Geometry: final body of the model. Coordinates: model frame, mm. Face numbers are marked on the shaded views. A direction names the side the tool comes from. Give positions to 0.01 mm unless a question says otherwise; leave off trailing zeros. Order: outer loops, then holes, each group sorted by start corner. A loop starts at its lowest first (then second) coordinate and runs counter-clockwise, first axis right, second up. Notation, with made-up numbers: (74, -12) -> (107, -12) arc R22 ccw to (107, 20) -> close; hole circle Ø6 at (29, -26). An arc over 180 degrees is marked (long way). Answer in a Markdown table with one row per item. Add a question column.
Q1. Contact query for flat-ended pins moving along their axis: P1, Ø6.5, axis at y = -132, z = 4.5, coming from the -X side; P2, Ø6, axis at x = 420.5, z = -61.5, coming from the +Y side; P3, Ø9, axis at y = -115, z = 4.5, coming from the +X side. Output: stop coordinate, or through.
Q2. Cut plane A-A on z = -26. Return the cut outline in (x, y).
Q3. Cut plane D-D on y = -129.5. Return the cut outline in (x, z), and give its area (3 significant figures).
Q4. Cut plane B-B on x = 380. Return the cut outline in (y, z), and give its area (3 significant figures).
Q5. Set-up query: the marked faces 1 and 2. Return all of +Z, -Z, +X, -X, +Y, -Y with unobstructed straight access to the full face (end or side cutting, diameter ignored); none if empty.
Q6. Cut plane C-C on y = -81. Return the cut outline in (x, z), and give its area (3 significant figures).
Q7. Line query: line 1 along X through (y, z) = (-82, -13); line 2 along Y through (x, z) = (322, -4.5); line 3 along Z through (x, y) = (51.5, -206.5). Output: solid intervals per line, ascending. Write a range as from..to.
Q8. Pull-direction query (Y, two-part tool) for the marked faces 3, 4, 5 and 6; classes: +Y half, -Y half, draft (parallel to the pull), parting line (faces both ways), or undercut.
Autodesk Inventor part; units mm, degrees
ref_plane "YZ Plane" through (0, 0, 0) normal (1, 0, 0) x (0, 1, 0)
ref_plane "XZ Plane" through (0, 0, 0) normal (0, 1, 0) x (-1, 0, 0)
ref_plane "XY Plane" through (0, 0, 0) normal (0, 0, 1) x (1, 0, 0)
sketch "Sketch1" plane through (0, 0, 0) normal (0, 0, 1) x (1, 0, 0)
  line L0 (-17.8746, 7.514) -> (482.1254, 7.514)
  line L1 (482.1254, 7.514) -> (482.1254, -242.486)
  line L2 (482.1254, -242.486) -> (-17.8746, -242.486)
  line L3 (-17.8746, -242.486) -> (-17.8746, 7.514)
  point P0 (0, 0)
  dimension "d0" = 500
  dimension "d1" = 250
extrude "Extrusion1" add sketch "Sketch1" along normal blind 8
sketch "Sketch2" plane through (0, 0, 0) normal (0, 0, -1) x (-1, 0, 0)
  point P0 (0, 0)
sketch "Sketch3" plane through (0, 0, 0) normal (0, 0, -1) x (-1, 0, 0)
  line L0 (17.8746, 7.514) -> (17.8746, -242.486)
  line L1 (0, -89.2163) -> (17.8746, -89.2163)
  line L2 (17.8746, -89.2163) -> (17.8746, -180.8626)
  line L3 (17.8746, -180.8626) -> (0, -180.8626)
  line L4 (0, -180.8626) -> (0, -89.2163)
  line L5 (-482.1254, -242.486) -> (-482.1254, 7.514)
  line L6 (-465.1744, -89.2163) -> (-482.1254, -89.2163)
  line L7 (-482.1254, -89.2163) -> (-482.1254, -180.8626)
  line L8 (-482.1254, -180.8626) -> (-465.1744, -180.8626)
  line L9 (-465.1744, -180.8626) -> (-465.1744, -89.2163)
  point P0 (0, 0)
extrude "Extrusion2" cut sketch "Sketch3" against normal blind 8
sketch "Sketch4" plane through (0, 0, 0) normal (0, 0, -1) x (-1, 0, 0)
  line L0 (17.8746, -89.2163) -> (17.8746, 7.514)
  line L1 (17.8746, -73.5948) -> (-191.2332, -73.5948)
  line L2 (-191.2332, -73.5948) -> (-191.2332, -89.2163)
  line L3 (-191.2332, -89.2163) -> (17.8746, -89.2163)
  line L4 (17.8746, -89.2163) -> (17.8746, -73.5948)
  line L5 (17.8746, -180.8626) -> (0, -180.8626)
  line L6 (17.8746, -180.8626) -> (-191.2332, -180.8626)
  line L7 (-191.2332, -180.8626) -> (-191.2332, -196.8404)
  line L8 (-191.2332, -196.8404) -> (17.8746, -196.8404)
  line L9 (17.8746, -196.8404) -> (17.8746, -180.8626)
  line L10 (-482.1254, 7.514) -> (-482.1254, -89.2163)
  line L11 (-482.1254, -89.2163) -> (-286.3362, -89.2163)
  line L12 (-286.3362, -89.2163) -> (-286.3362, -73.5948)
  line L13 (-286.3362, -73.5948) -> (-482.1254, -73.5948)
  line L14 (-482.1254, -73.5948) -> (-482.1254, -89.2163)
  line L15 (-482.1254, -180.8626) -> (-482.1254, -242.486)
  line L16 (-286.3362, -180.8626) -> (-482.1254, -180.8626)
  line L17 (-482.1254, -180.8626) -> (-482.1254, -196.8404)
  line L18 (-482.1254, -196.8404) -> (-286.3362, -196.8404)
  line L19 (-286.3362, -196.8404) -> (-286.3362, -180.8626)
  point P0 (0, 0)
extrude "Extrusion3" add sketch "Sketch4" along normal blind 76.2
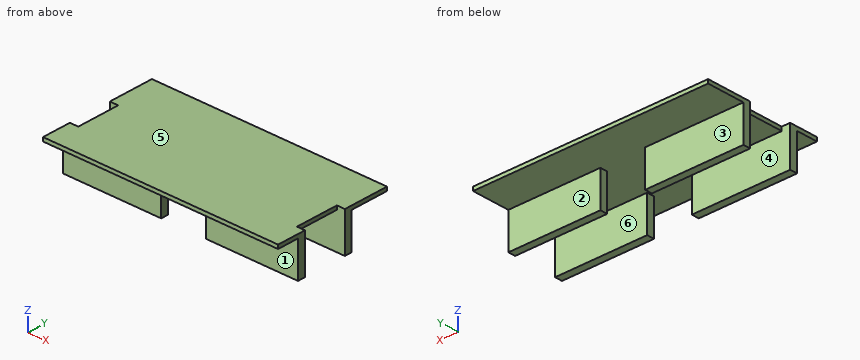
Completed:
| question | item | result |
|---|---|---|
| 1 | P1 | stops at x = 0 |
| 1 | P2 | stops at y = -73.59 |
| 1 | P3 | stops at x = 465.17 |
| 2 | outline | (-17.87, -196.84) -> (191.23, -196.84) -> (191.23, -180.86) -> (-17.87, -180.86) -> close; (-17.87, -89.22) -> (191.23, -89.22) -> (191.23, -73.59) -> (-17.87, -73.59) -> close; (286.34, -196.84) -> (482.13, -196.84) -> (482.13, -180.86) -> (286.34, -180.86) -> close; (286.34, -89.22) -> (482.13, -89.22) -> (482.13, -73.59) -> (286.34, -73.59) -> close |
| 3 | outline | (0, 0) -> (465.17, 0) -> (465.17, 8) -> (0, 8) -> close |
| 3 | area | 3,720 mm² |
| 4 | outline | (-242.49, 0) -> (-196.84, 0) -> (-196.84, -76.2) -> (-180.86, -76.2) -> (-180.86, 0) -> (-89.22, 0) -> (-89.22, -76.2) -> (-73.59, -76.2) -> (-73.59, 0) -> (7.51, 0) -> (7.51, 8) -> (-242.49, 8) -> close |
| 4 | area | 4,410 mm² |
| 5 | face 1 | -Z, +X, -X, -Y |
| 5 | face 2 | -Z, +X, -X, +Y |
| 6 | outline | (-17.87, -76.2) -> (191.23, -76.2) -> (191.23, 0) -> (286.34, 0) -> (286.34, -76.2) -> (482.13, -76.2) -> (482.13, 8) -> (-17.87, 8) -> close |
| 6 | area | 34,900 mm² |
| 7 | line 1 | x = -17.87..191.23, 286.34..482.13 |
| 7 | line 2 | y = -196.84..-180.86, -89.22..-73.59 |
| 7 | line 3 | z = 0..8 |
| 8 | face 3 | +Y half |
| 8 | face 4 | undercut |
| 8 | face 5 | draft |
| 8 | face 6 | undercut |
